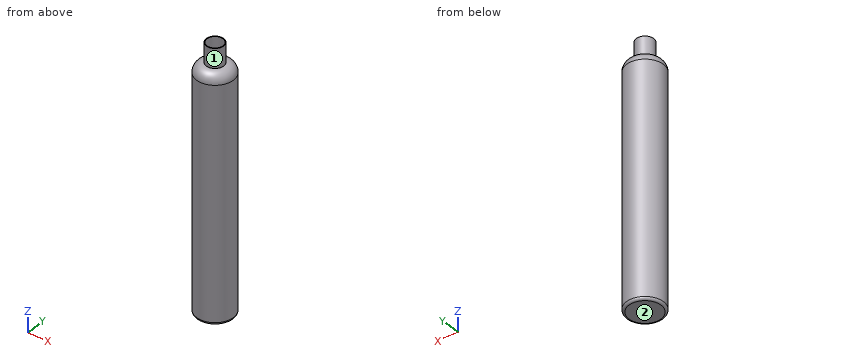
from build123d import *

# Parameters (mm, degrees)
F0_R     = 114.5
F1_DEPTH = 1500
F2_R     = 60
F3_R     = 15
F4_R     = 54.5
F4_R_2   = 50
F5_DEPTH = 120


with BuildPart() as f1:
    # F0 (on Top) → F1 (new body)
    with BuildSketch(Plane.XY):
        Circle(F0_R)
    extrude(amount=F1_DEPTH)

    # F2
    f2_edges = [f1.edges().sort_by_distance(p)[0] for p in [
        (-114.5, 0, 1500),
    ]]
    fillet(f2_edges, radius=F2_R)

    # F3
    f3_edges = [f1.edges().sort_by_distance(p)[0] for p in [
        (-114.5, 0, 0),
    ]]
    fillet(f3_edges, radius=F3_R)

    # F4 (on face) → F5 (join)
    with BuildSketch(Plane.XY.offset(1500)):
        Circle(F4_R)
        Circle(F4_R_2, mode=Mode.SUBTRACT)
    extrude(amount=F5_DEPTH)


solid = f1.part
Geometry: final body of the model. Coordinates: model frame, mm. Face numbers are marked on the shaded views. A direction names the side the tool comes from. Round coordinates to 2 decimals unless told otherwise and drop trailing zeros. Order: outer loops, then holes, each group sorted by start corner. A loop starts at its lowest first (then second) coordinate and runs counter-clockwise, first axis right, second up.
Q1. Material intervals for probe 1 along Y at (x, z) = (0, 1540); probe 2 along Z at (x, y) = (-42.5, 2); probe 3 along Y at (x, z) = (-55, 723.5), sorted ascending.
Result sheet:
probe 1: y = -54.5 to -50, 50 to 54.5
probe 2: z = 0 to 1500
probe 3: y = -100.43 to 100.43
Q2. Pin query (flat end, axial travel): pin 1 (10 mm diameter, centred on x = -13.5, y = 26, fed in from +Z); pin 2 (1.5 mm diameter, centred on y = -82, z = 665, fed in from +X); pin 3 (10 mm diameter, centred on x = 74.5, y = 65, fed in from -Z); pin 4 (12 mm diameter, centred on x = 70.5, z = 208, fed in from +Y). Return the tip coordinate at first contact, or that it passes through.
Result sheet:
pin 1: stops at z = 1500
pin 2: stops at x = 80.68
pin 3: stops at z = 0
pin 4: stops at y = 94.6
Q3. Section A-A, the plane z = 982.5. Output: boundary loops of the cut face in (x, y).
Result sheet:
outline: circle Ø229 at (0, 0)
Q4. Access query for the marked faces 1 and 2. Directions: +Z, -Z, +X, -X, +Y, -Y. A direction counts if a zero-diameter tool reaches every point of the face in a straight line with its end or side. Return the directions, or none.
Result sheet:
face 1: +Z
face 2: -Z, +X, -X, +Y, -Y
